Here's how the part is built. I have some questions about the finished solid (model axes, mm). A direction names the side the tool comes from. Give positions to 0.01 mm unless a question says otherwise; leave off trailing zeros. Write each loop counter-clockwise with the first axis right and the second up, starting at its lowest first coordinate (ties: lowest second). Pieces come first, ordered by that corner, then holes. Notation, with made-up numbers: (23.25, 23) - (43.25, 23) arc R36 cw to (43.25, 57) - close; hole circle Ø2 at (39.25, 26.5). An arc over 180 degrees is marked (long way). Write each question's results on one line, items separated by ' | '. Start each with the question number.
Item 1: We'd pull the mould along Y, two halves only. Please class faces 1 (the flat face through (0, 0, 0)), 2 (the flat face through (-0.408, 2.385, 26.688)), 3 (the cylindrical face through (-0.69, -3.1, 12.52)): +Y half, -Y half, draft (parallel to the pull), parting line (faces both ways), or undercut.
Item 2: Which directions (+Z, -Z, +X, -X, +Y, -Y) give clear straight access to the entire face, cutting with the end or side of a thin tool? Please do faces 4 (the flat face through (1.9, 1.5, 26.7)), 5 (the flat face through (-0.1, -3.5, 25.4)).
Item 3: Please list where these lines run through material, in increasing order: line 1 along Y through (x, z) = (0, 17.75) (3 decimals); line 2 along Z through (x, y) = (-1.25, 1.25); line 3 along Y through (x, z) = (1.5, 24).
Item 4: Suppose I cut it at A-A on z = 18.25. List the corners of the cut face in (x, y) for me (3 decimals).
Item 5: Will these pins go through, and if not, where does the flat tip stop? P1, Ø3, axis at y = 3.5, z = 22, coming from the -X side; P2, Ø3, axis at y = 2, z = 12.5, coming from the +X side; P3, Ø5, axis at y = -3.5, z = 25, coming from the +X side.
```python
from build123d import *

# Parameters (mm, degrees)
SKETCH1_R           = 3.175
BOSS_EXTRUDE1_DEPTH = 25.4
SKETCH2_R           = 5.334
BOSS_EXTRUDE2_DEPTH = 2.54
FILLET3_R           = 2.54
CUT_EXTRUDE2_DEPTH  = 2.54


with BuildPart() as part:
    # Sketch1 → Boss-Extrude1 (new body)
    with BuildSketch(Plane.XY):
        Circle(SKETCH1_R)
    extrude(amount=BOSS_EXTRUDE1_DEPTH)

    # Sketch2 → Boss-Extrude2 (add)
    with BuildSketch(Plane.XY.offset(25.4)):
        Circle(SKETCH2_R)
    extrude(amount=BOSS_EXTRUDE2_DEPTH)

    # Fillet3
    fillet3_edges = [part.edges().sort_by_distance(p)[0] for p in [
        (-5.334, 0, 27.94),
    ]]
    fillet(fillet3_edges, radius=FILLET3_R - 0.0001)  # a hair under: the kernel refuses the full size

    # Sketch6 → Cut-Extrude2 (cut)
    with BuildSketch(Plane.XY.offset(27.94)):
        Polygon((1.802599016, -2.134730144), (2.750030043, 0.493731468), (0.947431027, 2.628461612), (-1.802599016, 2.134730144), (-2.750030043, -0.493731468), (-0.947431027, -2.628461612), align=None)
    extrude(amount=-CUT_EXTRUDE2_DEPTH, mode=Mode.SUBTRACT)


solid = part.part
```
Checked values:
1) face 1: draft | face 2: undercut | face 3: parting line
2) face 4: +Z | face 5: -Z
3) line 1: y = -3.175 to 3.175 | line 2: z = 0 to 25.4 | line 3: y = -2.8 to 2.8
4) outline: circle Ø6.35 at (0, 0)
5) P1: stops at x = -2.47 | P2: stops at x = 3.14 | P3: stops at x = 5.23
